from build123d import *

# Parameters (mm, degrees)
SKETCH1_R           = 8
BOSS_EXTRUDE1_DEPTH = 10
BOSS_EXTRUDE2_DEPTH = 10
SKETCH3_R           = 4.5
BOSS_EXTRUDE3_DEPTH = 7
SKETCH3_2_R         = 4.5
BOSS_EXTRUDE4_DEPTH = 7
BOSS_EXTRUDE5_START = 7
SKETCH4_R           = 4.5
BOSS_EXTRUDE5_DEPTH = 7
SKETCH5_R           = 3
CUT_EXTRUDE9_DEPTH  = 7


with BuildPart() as part:
    # Sketch1 → Boss-Extrude1 (new body)
    with BuildSketch(Plane.XY):
        Circle(SKETCH1_R)
    extrude(amount=BOSS_EXTRUDE1_DEPTH)

    # Sketch2 → Boss-Extrude2 (add)
    with BuildSketch(Plane.XY.offset(10)):
        Polygon((-1, 7.937253933), (-0.5, 10.937253933), (0.5, 10.937253933), (1, 7.937253933), align=None)
        Polygon((2.314826562, 7.65777892), (3.99180922, 10.195046971), (4.905354678, 9.788310328), (4.141917478, 6.844305634), align=None)
        Polygon((5.229398583, 6.054204363), (7.793398362, 7.690023769), (8.462528969, 6.946878943), (6.567659795, 4.567914712), align=None)
        Polygon((7.23976008, 3.40380287), (10.247438126, 3.855325595), (10.556455121, 2.904269079), (7.857794069, 1.501689838), align=None)
        Polygon((7.998301289, 0.164852939), (10.929602743, -0.645993398), (10.82507428, -1.640515294), (7.789244362, -1.824190852), align=None)
        Polygon((7.373863542, -3.102601563), (9.721939754, -5.035614265), (9.221939754, -5.901639668), (6.373863542, -4.83465237), align=None)
        Polygon((5.4744178, -5.833588068), (6.83326506, -8.554531678), (6.024248065, -9.14231693), (3.856383811, -7.009158573), align=None)
        Polygon((2.628395486, -7.5558942), (2.763056759, -10.594292848), (1.784909158, -10.802204539), (0.672100285, -7.971717582), align=None)
        Polygon((-0.672100285, -7.971717582), (-1.784909158, -10.802204539), (-2.763056759, -10.594292848), (-2.628395486, -7.5558942), align=None)
        Polygon((-3.856383811, -7.009158573), (-6.024248065, -9.14231693), (-6.83326506, -8.554531678), (-5.4744178, -5.833588068), align=None)
        Polygon((-6.373863542, -4.83465237), (-9.221939754, -5.901639668), (-9.721939754, -5.035614265), (-7.373863542, -3.102601563), align=None)
        Polygon((-7.789244362, -1.824190852), (-10.82507428, -1.640515294), (-10.929602743, -0.645993398), (-7.998301289, 0.164852939), align=None)
        Polygon((-7.857794069, 1.501689838), (-10.556455121, 2.904269079), (-10.247438126, 3.855325595), (-7.23976008, 3.40380287), align=None)
        Polygon((-6.567659795, 4.567914712), (-8.462528969, 6.946878943), (-7.793398362, 7.690023769), (-5.229398583, 6.054204363), align=None)
        Polygon((-4.141917478, 6.844305634), (-4.905354678, 9.788310328), (-3.99180922, 10.195046971), (-2.314826562, 7.65777892), align=None)
    extrude(amount=-BOSS_EXTRUDE2_DEPTH)

    # Sketch3 → Boss-Extrude3 (add)
    with BuildSketch(Plane.XY.offset(10)):
        Circle(SKETCH3_R)
    extrude(amount=BOSS_EXTRUDE3_DEPTH)

    # Sketch3<2> → Boss-Extrude4 (add)
    with BuildSketch(Plane.XY.offset(10)):
        Circle(SKETCH3_2_R)
    extrude(amount=BOSS_EXTRUDE4_DEPTH)

    # Sketch4 → Boss-Extrude5 (add)
    with BuildSketch(Plane(origin=(0, 0, 0), x_dir=(-1, 0, 0), z_dir=(0, 0, -1)).offset(BOSS_EXTRUDE5_START)):
        with Locations(Location((0, 0, 0), (0, 0, 180))):
            Circle(SKETCH4_R)
    extrude(amount=-BOSS_EXTRUDE5_DEPTH)

    # Sketch5 → Cut-Extrude9 (cut)
    with BuildSketch(Plane(origin=(0, 0, -7), x_dir=(-1, 0, 0), z_dir=(0, 0, -1))):
        Circle(SKETCH5_R)
    extrude(amount=-CUT_EXTRUDE9_DEPTH, mode=Mode.SUBTRACT)


solid = part.part
Input: part model. Units: mm. Frame: model coordinates. A direction names the side the tool comes from. Round coordinates to 2 decimals unless told otherwise and drop trailing zeros. Loops run counter-clockwise (first coordinate to the right, second up) from the corner with the lowest first, then second, coordinate; pieces in that order, holes last. Notation, with made-up numbers: M 29.5,27 L 85.5,27 A21 ccw 85.5,56 Z; hole C 39.25,-0.5 d2. An arc over 180 degrees is marked long. Answer as CSV lines item,"result". Start each with the question number.
(1) Section D-D, the plane y = 0.5. Output: boundary loops of the cut face in (x, z).
(2) Line query: line 1 (Y direction, x = 0, z = -4.75); line 2 (Z direction, x = -4.5, y = -7); line 3 (Y direction, x = -8.75, z = 2.25). Output: solid intervals per line, ascending. Write a range as [from, to].
(3) Reachability of faces 1 (the flat face through (8.531, -4.056, 5.07)), 2 (the flat face through (3.142, 8.909, 5.07)), 3 (the flat face through (0, -5, 0)) from +Z, -Z, +X, -X, +Y, -Y: full face, straight path, thin tool, end or side. Return the list, or none.
(4) First-contact query: pin 1 (1 mm diameter, centred on x = 0.5, y = 7.5, fed in from -Z); pin 2 (11 mm diameter, centred on x = -0.5, y = -2, fed in from -Z); pin 3 (12 mm diameter, centred on x = 7, z = 10, fed in from +Y); pin 4 (1.5 mm diameter, centred on x = 8.5, z = 7.5, fed in from +Y). Flat tips, straight axial feed; report the tip coordinate or a pass-through.
(5) Draft query along X for faces 4 (the flat face through (0, 10.937, 5)), 5 (the cylindrical face through (0, -8, 5)), 6 (the flat face through (-8.56, -4.08, 5.07)). Return one class per face: released by +X, released by -X, zero draft, split by the parting line, or undercut.
(6) Section B-B, the plane y = -5.5. Output: boundary loops of the cut face in (x, z), plus the area to 3 significant figures.
(7) Section A-A, the plane x = 0. Output: boundary loops of the cut face in (y, z).
(8) Section C-C, the plane z = 13. Output: boundary loops of the cut face in (x, y).
Values found:
1,outline,"M -7.98,0 L -4.47,0 L -4.47,-7 L -2.96,-7 L -2.96,0 L 2.96,0 L 2.96,-7 L 4.47,-7 L 4.47,0 L 7.98,0 L 7.98,10 L 4.47,10 L 4.47,17 L -4.47,17 L -4.47,10 L -7.98,10 Z"
2,line 1,"y = [-4.5, -3], [3, 4.5]"
2,line 2,"z = [0, 10]"
2,line 3,"y = [-5.72, -4.24], [-1.77, -0.04], [1.97, 3.63]"
3,face 1,"+Z, -Z, +X"
3,face 2,"+Z, -Z, +Y"
3,face 3,"-Z"
4,pin 1,"stops at z = 0"
4,pin 2,"stops at z = -7"
4,pin 3,"stops at y = 10.2"
4,pin 4,"stops at y = 7.69"
5,face 4,"zero draft"
5,face 5,"undercut"
5,face 6,"released by -X"
6,outline,"M -9.45,0 L -8.15,0 L -8.15,10 L -9.45,10 Z; M -5.81,0 L 5.81,0 L 5.81,10 L -5.81,10 Z; M 8.15,0 L 9.45,0 L 9.45,10 L 8.15,10 Z"
6,area,"142 mm²"
7,outline,"M -8,0 L -4.5,0 L -4.5,-7 L -3,-7 L -3,0 L 3,0 L 3,-7 L 4.5,-7 L 4.5,0 L 10.94,0 L 10.94,10 L 4.5,10 L 4.5,17 L -4.5,17 L -4.5,10 L -8,10 Z"
8,outline,"C 0,0 d9"
